Design review of the part built by this model. Coordinates are the model's own, in mm. Give positions to 0.01 mm unless a question says otherwise; leave off trailing zeros. One line per item, written item: value.
from build123d import *

# Parameters (mm, degrees)
BOSS_EXTRUDE1_DEPTH = 5
FILLET2_R           = 1
SKETCH5_R           = 10.3
CUT_EXTRUDE1_DEPTH  = 0.5
CHAMFER1_SIZE       = 0.5
SKETCH6_OUTSIDE_W   = 384.304
SKETCH6_OUTSIDE_H   = 383.29
SKETCH6_OUTSIDE_R   = 12.75
CUT_EXTRUDE2_DEPTH  = 100.2
CUT_EXTRUDE2_DRAFT  = -60
SKETCH7_OUTSIDE_W   = 177.498
SKETCH7_OUTSIDE_H   = 176.484
SKETCH7_OUTSIDE_R   = 12.75
CUT_EXTRUDE3_DEPTH  = 40.5
CUT_EXTRUDE3_DRAFT  = -60
CUT_EXTRUDE4_DEPTH  = 40.5
SKETCH9_R           = 11.4
SKETCH9_R_2         = 5.625
CUT_EXTRUDE5_DEPTH  = 3.4
SKETCH10_R          = 6
CUT_EXTRUDE6_DEPTH  = 1


with BuildPart() as part:
    # Sketch1 → Boss-Extrude1 (new body)
    with BuildSketch(Plane(origin=(0, 0, 0), x_dir=(1, 0, 0), z_dir=(0, 1, 0))):
        with BuildLine():
            ThreePointArc((0, 11), (4.248983673, 13.077027099), (6.465637775, 8.899186938))
            ThreePointArc((6.465637775, 8.899186938), (11.123983673, 8.082047219), (10.461621679, 3.399186938))
            ThreePointArc((10.461621679, 3.399186938), (13.75, 0), (10.461621679, -3.399186938))
            ThreePointArc((10.461621679, -3.399186938), (11.123983673, -8.082047219), (6.465637775, -8.899186938))
            ThreePointArc((6.465637775, -8.899186938), (4.248983673, -13.077027099), (0, -11))
            ThreePointArc((0, -11), (-4.248983673, -13.077027099), (-6.465637775, -8.899186938))
            ThreePointArc((-6.465637775, -8.899186938), (-11.123983673, -8.082047219), (-10.461621679, -3.399186938))
            ThreePointArc((-10.461621679, -3.399186938), (-13.75, 0), (-10.461621679, 3.399186938))
            ThreePointArc((-10.461621679, 3.399186938), (-11.123983673, 8.082047219), (-6.465637775, 8.899186938))
            ThreePointArc((-6.465637775, 8.899186938), (-4.248983673, 13.077027099), (0, 11))
        make_face()
    extrude(amount=BOSS_EXTRUDE1_DEPTH)

    # Fillet2
    fillet2_edges = [part.edges().sort_by_distance(p)[0] for p in [
        (10.461621679, 2.5, -3.399186938),
        (10.461621679, 2.5, 3.399186938),
        (6.465637775, 2.5, 8.899186938),
        (0, 2.5, 11),
        (-6.465637775, 2.5, 8.899186938),
        (-10.461621679, 2.5, 3.399186938),
        (-10.461621679, 2.5, -3.399186938),
        (-6.465637775, 2.5, -8.899186938),
        (0, 2.5, -11),
        (6.465637775, 2.5, -8.899186938),
    ]]
    fillet(fillet2_edges, radius=FILLET2_R)

    # Sketch5 → Cut-Extrude1 (cut)
    with BuildSketch(Plane(origin=(0, 5, 0), x_dir=(1, 0, 0), z_dir=(0, 1, 0))):
        with Locations(Location((0, 0, 0), (0, 0, 270))):
            Circle(SKETCH5_R)
    extrude(amount=-CUT_EXTRUDE1_DEPTH, mode=Mode.SUBTRACT)

    # Chamfer1
    chamfer1_edges = [part.edges().sort_by_distance(p)[0] for p in [
        (0, 5, -10.3),
    ]]
    chamfer(chamfer1_edges, length=CHAMFER1_SIZE - 0.0001)  # a hair under: the kernel refuses the full size


with BuildPart() as cut_extrude2_tool:
    # Sketch6 outside → Cut-Extrude2 (with draft: the straight prism first)
    with BuildSketch(Plane(origin=(0, 5, 0), x_dir=(1, 0, 0), z_dir=(0, 1, 0))):
        Rectangle(SKETCH6_OUTSIDE_W, SKETCH6_OUTSIDE_H)
        Circle(SKETCH6_OUTSIDE_R, mode=Mode.SUBTRACT)
    extrude(amount=-CUT_EXTRUDE2_DEPTH)
    # Cut-Extrude2: the draft: its side faces are tilted about the plane it starts from
    cut_extrude2_sides = [cut_extrude2_tool.faces().sort_by_distance(p)[0] for p in [
        (0, -45.1, 191.645),
        (192.152, -45.1, 0),
        (0, -45.1, -191.645),
        (-192.152, -45.1, 0),
        (-12.75, -45.1, 0),
    ]]
    draft(cut_extrude2_sides, Plane(origin=(0, 5, 0), x_dir=(1, 0, 0), z_dir=(0, 1, 0)), CUT_EXTRUDE2_DRAFT)


with BuildPart() as part_1:
    add(part.part)

    # Cut-Extrude2: cut by cut_extrude2_tool
    add(cut_extrude2_tool.part, mode=Mode.SUBTRACT)


with BuildPart() as cut_extrude3_tool:
    # Sketch7 outside → Cut-Extrude3 (with draft: the straight prism first)
    with BuildSketch(Plane.XZ):
        Rectangle(SKETCH7_OUTSIDE_W, SKETCH7_OUTSIDE_H)
        Circle(SKETCH7_OUTSIDE_R, mode=Mode.SUBTRACT)
    extrude(amount=-CUT_EXTRUDE3_DEPTH)
    # Cut-Extrude3: the draft: its side faces are tilted about the plane it starts from
    cut_extrude3_sides = [cut_extrude3_tool.faces().sort_by_distance(p)[0] for p in [
        (0, 20.25, -88.242),
        (88.749, 20.25, 0),
        (0, 20.25, 88.242),
        (-88.749, 20.25, 0),
        (-12.75, 20.25, 0),
    ]]
    draft(cut_extrude3_sides, Plane.XZ, CUT_EXTRUDE3_DRAFT)


with BuildPart() as part_2:
    add(part_1.part)

    # Cut-Extrude3: cut by cut_extrude3_tool
    add(cut_extrude3_tool.part, mode=Mode.SUBTRACT)

    # Sketch8 → Cut-Extrude4 (cut)
    with BuildSketch(Plane(origin=(0, 4.5, 0), x_dir=(1, 0, 0), z_dir=(0, 1, 0))):
        with BuildLine():
            Line((-2.65, -3.128498042), (-2.65, 3.128498042))
            ThreePointArc((-2.65, 3.128498042), (0, 4.1), (2.65, 3.128498042))
            Line((2.65, 3.128498042), (2.65, -3.128498042))
            ThreePointArc((2.65, -3.128498042), (0, -4.1), (-2.65, -3.128498042))
        make_face()
    extrude(amount=-CUT_EXTRUDE4_DEPTH, mode=Mode.SUBTRACT)

    # Sketch9 → Cut-Extrude5 (cut)
    with BuildSketch(Plane.XZ):
        with Locations(Location((0, 0, 0), (0, 0, 270))):
            Circle(SKETCH9_R)
        with Locations(Location((0, 0, 0), (0, 0, 270))):
            Circle(SKETCH9_R_2, mode=Mode.SUBTRACT)
    extrude(amount=-CUT_EXTRUDE5_DEPTH, mode=Mode.SUBTRACT)

    # Sketch10 → Cut-Extrude6 (cut)
    with BuildSketch(Plane.XZ):
        Circle(SKETCH10_R)
    extrude(amount=-CUT_EXTRUDE6_DEPTH, mode=Mode.SUBTRACT)


solid = part_2.part
Item 1: To check wall thickness, follow line 1 along X through (y, z) = (1.7, 0) (3 decimals); line 2 along X through (y, z) = (0.8, 0); line 3 along Z through (x, y) = (2, 3). State the ranges of each line that lie inside material, in increasing order. Write a range as from..to.
Returned:
line 1: -13.75..-11.4, -5.625..-2.65, 2.65..5.625, 11.4..13.75
line 2: -13.75..-11.4, 11.4..13.75
line 3: -13.03..-11.22, -5.26..-3.58, 3.58..5.26, 11.22..13.03
Item 2: Clearance check with flat-ended pins moving along their axes: P1, Ø1.5, axis at x = -9, y = 1, coming from the +Z side; P2, Ø1, axis at x = 2, y = 2, coming from the -Z side; P3, Ø1, axis at y = 2, z = -0.5, coming from the +X side; P4, Ø6, axis at x = 1, z = 2.5, coming from the +Y side. State where each tip first meets the part, or that it passes through.
Returned:
P1: z = 9.48
P2: z = -13.17
P3: x = 13.75
P4: y = 4.5
Item 3: Draft analysis for pull direction Z (two halves, no side actions). For faces 1 (the flat face through (5, 3.4, 3)), 2 (the conical face through (-4.09, 0.22, -12.48)), 3 (the conical face through (-10.647, 4.779, 7.687)), 4 (the flat face through (2.65, 3, 0)), state which applies: pulls with the +Z half, pulls with the -Z half, needs draft (parallel to the pull), parting line crosses it, or undercut.
Returned:
face 1: undercut
face 2: pulls with the -Z half
face 3: pulls with the +Z half
face 4: undercut
Item 4: Add section B-B on y = 2.85. Count the separate pieces of the cut face and the enclosed holes in it, plus the area to 3 significant figures.
Returned:
separate pieces: 2
enclosed holes: 2
area: 185 mm²
